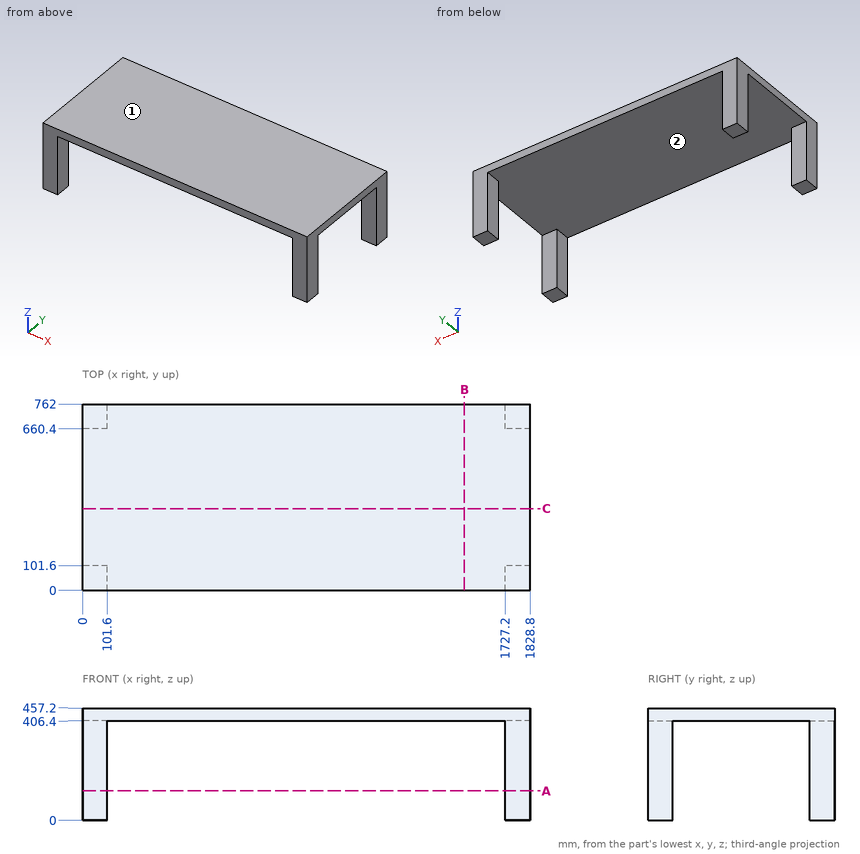
For this review, use the dimensioned drawing (mm, ordinates from the lowest corner) and the shaded views. Coordinates: 2 decimals unless noted, no trailing zeros. Order: outer loops, then holes, each group sorted by start corner. A loop starts at its lowest first (then second) coordinate and runs counter-clockwise, first axis right, second up. Notation, with made-up numbers: (61, 16) - (93, 16) arc R25 cw to (93, 30) - close; hole circle Ø2 at (-34.75, -13). An arc over 180 degrees is marked (long way). Answer in a Markdown table with one row per item.
(1) The part is to be moulded in two halves that separate along X. For the marked faces 1 and 2, say which applies: released by +X, released by -X, zero draft, split by the parting line, or undercut.
Checked values:
| item | result |
|---|---|
| face 1 | zero draft |
| face 2 | undercut |
(2) Consider section C-C on y = 334. State the section outline as (x, z) points, plus the area to 3 significant figures.
Checked values:
| item | result |
|---|---|
| outline | (0, 406.4) - (1828.8, 406.4) - (1828.8, 457.2) - (0, 457.2) - close |
| area | 92,900 mm^2 |
(3) Consider section B-B on x = 1560. State the section outline as (y, z) points.
Checked values:
| item | result |
|---|---|
| outline | (0, 406.4) - (762, 406.4) - (762, 457.2) - (0, 457.2) - close |
(4) Wall thickness on line 1 along X through (y, z) = (718.5, 313); line 2 along Z through (x, y) = (459.5, 39): over which ranges is each line inside the solid? List them lowest first. Write a range as from..to.
Checked values:
| item | result |
|---|---|
| line 1 | 0..101.6, 1727.2..1828.8 |
| line 2 | 406.4..457.2 |
(5) Consider section A-A on z = 120. State the section outline as (x, y) points, plus the area to 3 significant figures.
Checked values:
| item | result |
|---|---|
| outline | (0, 0) - (101.6, 0) - (101.6, 101.6) - (0, 101.6) - close; (0, 660.4) - (101.6, 660.4) - (101.6, 762) - (0, 762) - close; (1727.2, 0) - (1828.8, 0) - (1828.8, 101.6) - (1727.2, 101.6) - close; (1727.2, 660.4) - (1828.8, 660.4) - (1828.8, 762) - (1727.2, 762) - close |
| area | 41,300 mm^2 |
